The model under review builds one solid part; all positions refer to its coordinate system, in mm. A direction names the side the tool comes from. Give positions to 0.01 mm unless a question says otherwise; leave off trailing zeros. Order: outer loops, then holes, each group sorted by start corner. A loop starts at its lowest first (then second) coordinate and runs counter-clockwise, first axis right, second up.
```python
from build123d import *

# Parameters (mm, degrees)
BOSS_EXTRUDE1_DEPTH = 2
BOSS_EXTRUDE2_DEPTH = 2
SKETCH4_W           = 3
SKETCH4_H           = 36.44
BOSS_EXTRUDE3_DEPTH = 2
SKETCH5_W           = 113.22
SKETCH5_H           = 3
BOSS_EXTRUDE4_DEPTH = 2
CUT_EXTRUDE1_REACH  = 4
SKETCH6_R           = 1.2
CUT_EXTRUDE2_REACH  = 4
SKETCH10_R          = 1.5
SKETCH11_W          = 5
SKETCH11_H          = 10
BOSS_EXTRUDE6_DEPTH = 95
SKETCH12_W          = 10
SKETCH12_H          = 5
BOSS_EXTRUDE7_DEPTH = 60
CUT_EXTRUDE3_REACH  = 99
SKETCH13_R          = 4
SKETCH14_W          = 10
SKETCH14_H          = 10
BOSS_EXTRUDE8_DEPTH = 60
CUT_EXTRUDE4_REACH  = 4
SKETCH16_W          = 20
SKETCH16_H          = 60


with BuildPart() as part:
    # Sketch1 → Boss-Extrude1 (new body)
    with BuildSketch(Plane(origin=(0, 0, 0), x_dir=(1, 0, 0), z_dir=(0, 1, 0))):
        Polygon((-76.190879746, -68.876090608), (-65.066970355, -80), (65, -80), (75, -70), (75, -30), (42.284331493, 59.968088394), (-42.212099054, 59.968088394), (-76.190879746, -28.818652669), align=None)
    extrude(amount=BOSS_EXTRUDE1_DEPTH)

    # Sketch2 → Boss-Extrude2 (add)
    with BuildSketch(Plane(origin=(0, 2, 0), x_dir=(1, 0, 0), z_dir=(0, 1, 0))):
        Polygon((-75.066970355, -70), (75, -70), (70, -75), (-70.066970355, -75), align=None)
    extrude(amount=BOSS_EXTRUDE2_DEPTH)

    # Sketch4 → Boss-Extrude3 (add)
    with BuildSketch(Plane(origin=(0, 2, 0), x_dir=(1, 0, 0), z_dir=(0, 1, 0))):
        with Locations((-59.300879746, -51.78)):
            Rectangle(SKETCH4_W, SKETCH4_H)
    extrude(amount=BOSS_EXTRUDE3_DEPTH)

    # Sketch5 → Boss-Extrude4 (add)
    with BuildSketch(Plane(origin=(0, 2, 0), x_dir=(1, 0, 0), z_dir=(0, 1, 0))):
        with Locations((-1.190879746, -35.1)):
            Rectangle(SKETCH5_W, SKETCH5_H)
    extrude(amount=BOSS_EXTRUDE4_DEPTH)

    # Sketch6 → Cut-Extrude1 (cut, up to next)
    with BuildSketch(Plane(origin=(0, 2, 0), x_dir=(1, 0, 0), z_dir=(0, 1, 0)), mode=Mode.PRIVATE) as cut_extrude1_sk1:
        with Locations((-23.96388378, 31)):
            Circle(SKETCH6_R)
    cut_extrude1_tool1 = extrude(cut_extrude1_sk1.sketch, amount=-CUT_EXTRUDE1_REACH, mode=Mode.PRIVATE) & part.part
    add(cut_extrude1_tool1.solids().sort_by_distance((-23.963884, 2, -31))[0], mode=Mode.SUBTRACT)
    # Sketch6 → Cut-Extrude1 (cut, up to next)
    with BuildSketch(Plane(origin=(0, 2, 0), x_dir=(1, 0, 0), z_dir=(0, 1, 0)), mode=Mode.PRIVATE) as cut_extrude1_sk2:
        with Locations((24.03611622, 31)):
            Circle(SKETCH6_R)
    cut_extrude1_tool2 = extrude(cut_extrude1_sk2.sketch, amount=-CUT_EXTRUDE1_REACH, mode=Mode.PRIVATE) & part.part
    add(cut_extrude1_tool2.solids().sort_by_distance((24.036116, 2, -31))[0], mode=Mode.SUBTRACT)
    # Sketch6 → Cut-Extrude1 (cut, up to next)
    with BuildSketch(Plane(origin=(0, 2, 0), x_dir=(1, 0, 0), z_dir=(0, 1, 0)), mode=Mode.PRIVATE) as cut_extrude1_sk3:
        with Locations((-23.96388378, -27)):
            Circle(SKETCH6_R)
    cut_extrude1_tool3 = extrude(cut_extrude1_sk3.sketch, amount=-CUT_EXTRUDE1_REACH, mode=Mode.PRIVATE) & part.part
    add(cut_extrude1_tool3.solids().sort_by_distance((-23.963884, 2, 27))[0], mode=Mode.SUBTRACT)
    # Sketch6 → Cut-Extrude1 (cut, up to next)
    with BuildSketch(Plane(origin=(0, 2, 0), x_dir=(1, 0, 0), z_dir=(0, 1, 0)), mode=Mode.PRIVATE) as cut_extrude1_sk4:
        with Locations((24.03611622, -27)):
            Circle(SKETCH6_R)
    cut_extrude1_tool4 = extrude(cut_extrude1_sk4.sketch, amount=-CUT_EXTRUDE1_REACH, mode=Mode.PRIVATE) & part.part
    add(cut_extrude1_tool4.solids().sort_by_distance((24.036116, 2, 27))[0], mode=Mode.SUBTRACT)

    # Sketch10 → Cut-Extrude2 (cut, up to next)
    with BuildSketch(Plane(origin=(0, 2, 0), x_dir=(1, 0, 0), z_dir=(0, 1, 0)), mode=Mode.PRIVATE) as cut_extrude2_sk1:
        with Locations((-5.96388378, 47.968088394)):
            Circle(SKETCH10_R)
    cut_extrude2_tool1 = extrude(cut_extrude2_sk1.sketch, amount=-CUT_EXTRUDE2_REACH, mode=Mode.PRIVATE) & part.part
    add(cut_extrude2_tool1.solids().sort_by_distance((-5.963884, 2, -47.968088))[0], mode=Mode.SUBTRACT)
    # Sketch10 → Cut-Extrude2 (cut, up to next)
    with BuildSketch(Plane(origin=(0, 2, 0), x_dir=(1, 0, 0), z_dir=(0, 1, 0)), mode=Mode.PRIVATE) as cut_extrude2_sk2:
        with Locations((6.03611622, 47.968088394)):
            Circle(SKETCH10_R)
    cut_extrude2_tool2 = extrude(cut_extrude2_sk2.sketch, amount=-CUT_EXTRUDE2_REACH, mode=Mode.PRIVATE) & part.part
    add(cut_extrude2_tool2.solids().sort_by_distance((6.036116, 2, -47.968088))[0], mode=Mode.SUBTRACT)

    # Sketch11 → Boss-Extrude6 (add)
    with BuildSketch(Plane(origin=(0, 2, 0), x_dir=(1, 0, 0), z_dir=(0, 1, 0))):
        with Locations((-32.46388378, 32.968088394)):
            Rectangle(SKETCH11_W, SKETCH11_H)
        with Locations((32.53611622, 32.968088394)):
            Rectangle(SKETCH11_W, SKETCH11_H)
    extrude(amount=BOSS_EXTRUDE6_DEPTH)

    # Sketch12 → Boss-Extrude7 (add)
    with BuildSketch(Plane(origin=(-29.96388378, 0, 0), x_dir=(0, 0, -1), z_dir=(1, 0, 0))):
        with Locations((32.968088394, 94.5)):
            Rectangle(SKETCH12_W, SKETCH12_H)
    extrude(amount=BOSS_EXTRUDE7_DEPTH)

    # Sketch13 → Cut-Extrude3 (cut, up to next)
    with BuildSketch(Plane(origin=(0, 97, 0), x_dir=(1, 0, 0), z_dir=(0, 1, 0)), mode=Mode.PRIVATE) as cut_extrude3_sk1:
        with Locations((0.03611622, 52.704663647)):
            Circle(SKETCH13_R)
    cut_extrude3_tool1 = extrude(cut_extrude3_sk1.sketch, amount=-CUT_EXTRUDE3_REACH, mode=Mode.PRIVATE) & part.part
    add(cut_extrude3_tool1.solids().sort_by_distance((0.036116, 97, -52.704664))[0], mode=Mode.SUBTRACT)

    # Sketch14 → Boss-Extrude8 (add)
    with BuildSketch(Plane(origin=(-29.96388378, 0, 0), x_dir=(0, 0, -1), z_dir=(1, 0, 0))):
        with Locations((32.968088394, 52)):
            Rectangle(SKETCH14_W, SKETCH14_H)
    extrude(amount=BOSS_EXTRUDE8_DEPTH)

    # Sketch16 → Cut-Extrude4 (cut, up to next)
    with BuildSketch(Plane(origin=(0, 2, 0), x_dir=(1, 0, 0), z_dir=(0, 1, 0)), mode=Mode.PRIVATE) as cut_extrude4_sk1:
        with Locations((-16.550598938, 29.968088394)):
            Rectangle(SKETCH16_W, SKETCH16_H)
    cut_extrude4_tool1 = extrude(cut_extrude4_sk1.sketch, amount=-CUT_EXTRUDE4_REACH, mode=Mode.PRIVATE) & part.part
    add(cut_extrude4_tool1.solids().sort_by_distance((-16.550599, 2, -29.968088))[0], mode=Mode.SUBTRACT)


solid = part.part
```
Item 1: For faces 1 (the flat face through (-1, 2, 77)), 2 (the cylindrical face through (-0.83, 1.01, -48.8)), 3 (the flat face through (30.036, 74, -33)), 4 (the flat face through (-58.964, 0.986, -16.196)), 5 (the flat face through (-3, 56, -37.968)), list the 3-axis set-ups (+Z, -Z, +X, -X, +Y, -Y) from which the entire face can be reached by the end or side of a thin tool; tool diameter is ignored.
Values found:
face 1: +Z, +X, -X, +Y
face 2: +Y, -Y
face 3: +Z, -Z
face 4: -Z, -X, +Y, -Y
face 5: -Z, +X, -X, +Y
Item 2: For line 1 (Y direction, x = 22.5, z = -34.5); line 2 (Y direction, x = -14, z = 64); line 3 (X direction, y = 1, z = -31), list the stretches that pass through material, from the lowest coordinate up.
Values found:
line 1: y = 0 to 2, 47 to 57, 92 to 97
line 2: y = 0 to 2
line 3: x = -53.3 to -26.55, -6.55 to 22.84, 25.24 to 52.82
Item 3: Take a section at A-A (y = 10). Give the boundary of the cut face in (x, z).
Values found:
outline: (-34.96, -37.97) - (-29.96, -37.97) - (-29.96, -27.97) - (-34.96, -27.97) - close; (30.04, -37.97) - (35.04, -37.97) - (35.04, -27.97) - (30.04, -27.97) - close
Item 4: Take a section at D-D (x = 39). Give the boundary of the cut face in (y, z), and give its area (3 significant figures).
Values found:
outline: (0, -59.97) - (2, -59.97) - (2, 33.6) - (4, 33.6) - (4, 36.6) - (2, 36.6) - (2, 70) - (4, 70) - (4, 75) - (2, 75) - (2, 80) - (0, 80) - close
area: 296 mm2
Item 5: Take a section at C-C (z = -41). Give the boundary of the cut face in (x, y).
Values found:
outline: (-49.47, 0) - (-26.55, 0) - (-26.55, 2) - (-49.47, 2) - close; (-6.55, 0) - (49.18, 0) - (49.18, 2) - (-6.55, 2) - close
Item 6: Clearance check with flat-ended pins moving along their axes: pin 1 Ø2 at (y, z) = (63, -37.5) entering from +X; pin 2 Ø2 at (y, z) = (1.5, -23.5) entering from +X; pin 3 Ø12 at (x, z) = (-25.5, 7.5) entering from +Y. State where each tip first meets the part, or that it passes through.
Values found:
pin 1: stops at x = 35.04
pin 2: stops at x = 55.91
pin 3: stops at y = 2
Item 7: Draft analysis for pull direction X (two halves, no side actions). For faces 6 (the flat face through (-2, 0, 25)), 7 (the flat face through (0, 47, -33)), 8 (the flat face through (-34.964, 49, -33)), 9 (the flat face through (-29.964, 24, -33)), state which applies: released by +X, released by -X, zero draft, split by the parting line, or undercut.
Values found:
face 6: zero draft
face 7: undercut
face 8: released by -X
face 9: undercut
Item 8: Take a section at B-B (z = 46.5). Give the boundary of the cut face in (x, y), and give its area (3 significant figures).
Values found:
outline: (-76.19, 0) - (75, 0) - (75, 2) - (-57.8, 2) - (-57.8, 4) - (-60.8, 4) - (-60.8, 2) - (-76.19, 2) - close
area: 308 mm2
